Source: CAD feature listing. Evaluate the final solid. Frame: model axes, mm. Face numbers are marked on the shaded views. Give positions to 0.01 mm unless a question says otherwise; leave off trailing zeros. Order: outer loops, then holes, each group sorted by start corner. A loop starts at its lowest first (then second) coordinate and runs counter-clockwise, first axis right, second up. Notation, with made-up numbers: (36.25, 36.5) - (68.25, 36.5) arc R27 cw to (68.25, 67.5) - close; hole circle Ø1 at (-4, 69.25). An arc over 180 degrees is marked (long way). Use CSV: the item, a comma, the result in double quotes.
```python
from build123d import *

# Parameters (mm, degrees)
SKETCH_R    = 6.5
SKETCH_R_2  = 3
SKETCH_R_3  = 2.5
PAD_DEPTH   = 10
FILLET_R    = 1
FILLET001_R = 5
FILLET002_R = 10


with BuildPart() as part:
    # Sketch → Pad (new body)
    with BuildSketch(Plane.XY):
        Polygon((-25, 45), (55, 45), (55, -75), (35, -75), (35, -115), (-25, -115), align=None)
        with Locations((0, -85)):
            Circle(SKETCH_R, mode=Mode.SUBTRACT)
        with Locations((-10, -52)):
            Circle(SKETCH_R_2, mode=Mode.SUBTRACT)
        with Locations((40, -52)):
            Circle(SKETCH_R_2, mode=Mode.SUBTRACT)
        with Locations((40, 22)):
            Circle(SKETCH_R_2, mode=Mode.SUBTRACT)
        with Locations((-10, 22)):
            Circle(SKETCH_R_2, mode=Mode.SUBTRACT)
        with Locations((25, -80)):
            Circle(SKETCH_R_3, mode=Mode.SUBTRACT)
        with Locations((-18, -80)):
            Circle(SKETCH_R_3, mode=Mode.SUBTRACT)
        with BuildLine():
            ThreePointArc((-5, -6.244998), (8, 0), (-5, 6.244998))
            Line((-5, 6.244998), (-5, 10))
            ThreePointArc((-5, 10), (-7, 12), (-9, 10))
            Line((-9, 10), (-9, -10))
            ThreePointArc((-9, -10), (-7, -12), (-5, -10))
            Line((-5, -10), (-5, -6.244998))
        make_face(mode=Mode.SUBTRACT)
    extrude(amount=PAD_DEPTH)

    # Fillet
    fillet_edges = [part.edges().sort_by_distance(p)[0] for p in [
        (55, -75, 5),
        (55, 45, 5),
        (-25, 45, 5),
    ]]
    fillet(fillet_edges, radius=FILLET_R)

    # Fillet001
    fillet001_edges = [part.edges().sort_by_distance(p)[0] for p in [
        (35, -75, 5),
    ]]
    fillet(fillet001_edges, radius=FILLET001_R)

    # Fillet002
    fillet002_edges = [part.edges().sort_by_distance(p)[0] for p in [
        (35, -115, 5),
        (-25, -115, 5),
    ]]
    fillet(fillet002_edges, radius=FILLET002_R)


solid = part.part
```
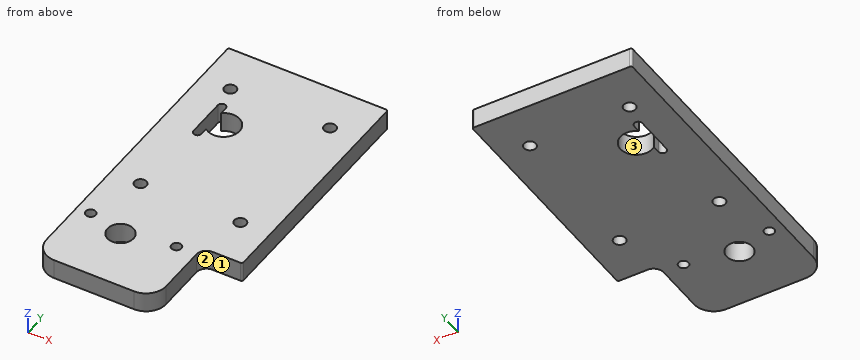
Item 1: Section C-C on z = 3. Count the separate pieces of the cut face and the enclosed holes in it, then the cut area to 3 significant figures.
Filled in:
separate pieces,"1"
enclosed holes,"8"
area,"11,400 mm2"
Item 2: Section B-B on x = 0. Return the cut outline in (y, z), then the cut area to 3 significant figures.
Filled in:
outline,"(-115, 0) - (-91.5, 0) - (-91.5, 10) - (-115, 10) - close; (-78.5, 0) - (-8, 0) - (-8, 10) - (-78.5, 10) - close; (8, 0) - (45, 0) - (45, 10) - (8, 10) - close"
area,"1,310 mm2"
Item 3: Mould query, pull axis X, two halves, no side actions, for the marked faces 1, 2 and 3. Classes: released by +X, released by -X, zero draft, split by the parting line, or undercut.
Filled in:
face 1,"zero draft"
face 2,"released by +X"
face 3,"undercut"
Item 4: Section D-D on x = -18. Return the cut outline in (y, z).
Filled in:
outline,"(-114.54, 0) - (-82.5, 0) - (-82.5, 10) - (-114.54, 10) - close; (-77.5, 0) - (45, 0) - (45, 10) - (-77.5, 10) - close"
Item 5: Material intervals for line 1 (Y direction, x = 0.5, z = 4); line 2 (Y direction, x = 5.5, z = 3.75); line 3 (X direction, y = -3, z = 5), sorted ascending. Write a range as from..to.
Filled in:
line 1,"y = -115..-91.48, -78.52..-7.98, 7.98..45"
line 2,"y = -115..-88.46, -81.54..-5.81, 5.81..45"
line 3,"x = -25..-9, 7.42..55"
Item 6: First-contact query: pin 1 (5.5 mm diameter, centred on x = -10, y = -52, fed in from -Z). Flat tip, straight axial feed; report the tip coordinate or a pass-through.
Filled in:
pin 1,"passes through"
Item 7: Section A-A on y = 22. Return the cut outline in (x, z), then the cut area to 3 significant figures.
Filled in:
outline,"(-25, 0) - (-13, 0) - (-13, 10) - (-25, 10) - close; (-7, 0) - (37, 0) - (37, 10) - (-7, 10) - close; (43, 0) - (55, 0) - (55, 10) - (43, 10) - close"
area,"680 mm2"
